```python
from build123d import *

# Parameters (mm, degrees)
PAD_DEPTH     = 16
SKETCH001_R   = 12
SKETCH001_R_2 = 15
POCKET_DEPTH  = 20


with BuildPart() as part:
    # Sketch → Pad (new body)
    with BuildSketch(Plane.YZ):
        Polygon((0, 0), (0, 116), (500, 116), (500, 0), (250, 0), align=None)
    extrude(amount=-PAD_DEPTH)

    # Sketch001 (on Face7 of Pad) → Pocket (cut)
    with BuildSketch(Plane(origin=(-16, 0, 0), x_dir=(0, -1, 0), z_dir=(-1, 0, 0))):
        with Locations((-215, 73.70748)):
            Circle(SKETCH001_R)
        with Locations((-285, 73.70748)):
            Circle(SKETCH001_R)
        with Locations((-450, 50)):
            Circle(SKETCH001_R_2)
        with Locations((-50, 50)):
            Circle(SKETCH001_R_2)
    extrude(amount=-POCKET_DEPTH, mode=Mode.SUBTRACT)


solid = part.part
```
Geometry check sheet. Reference: the model listing, model coordinates, mm. Give positions to 0.01 mm unless a question says otherwise; leave off trailing zeros. Order: outer loops, then holes, each group sorted by start corner. A loop starts at its lowest first (then second) coordinate and runs counter-clockwise, first axis right, second up. Notation, with made-up numbers: (-18.5, -23.75) -> (21.5, -23.75) arc R14 ccw to (21.5, -17.75) -> close; hole circle Ø10 at (73, 78.5). An arc over 180 degrees is marked (long way). Write each question's results on one line, items separated by ' | '. Start each with the question number.
(1) Gauge pin test, flat end, axial feed: P1, Ø18, axis at y = 450, z = 50, coming from the +X side. Record the tip position at first contact, or that the pin passes through.
(2) Scan lines: line 1 (Y direction, x = -14, z = 72.5); line 2 (Z direction, x = -12.5, y = 50); line 3 (Y direction, x = -7, z = 63). Record each from-to range of solid material in increasing order.
(3) Mould release check, pull along Y, two halves, no side actions. Record for faces 1 (the face through (-8.112, 461.056, 60.138)), 2 (the face through (-8, 500, 59)), 3 (the face through (-16, 253, 59)): pulls with the +Y half, pulls with the -Y half, needs draft (parallel to the pull), parting line crosses it, or undercut.
(4) Sectioned sample at D-D (y = 50). Enter the section's corners in (x, z).
(5) Sectioned sample at C-C (x = -11). Enter the section's corners in (y, z).
(6) Sectioned sample at A-A (z = 50). Enter the section's corners in (x, y).
(7) Sectioned sample at B-B (y = 215). Enter the section's corners in (x, z), plus the area to 3 significant figures.
Answer below:
1) P1: through
2) line 1: 0 to 203.06, 226.94 to 273.06, 296.94 to 500 | line 2: 0 to 35, 65 to 116 | line 3: 0 to 42.52, 57.48 to 209.58, 220.42 to 279.58, 290.42 to 442.52, 457.48 to 500
3) face 1: undercut | face 2: pulls with the +Y half | face 3: needs draft
4) outline: (-16, 0) -> (0, 0) -> (0, 35) -> (-16, 35) -> close; (-16, 65) -> (0, 65) -> (0, 116) -> (-16, 116) -> close
5) outline: (0, 0) -> (500, 0) -> (500, 116) -> (0, 116) -> close; hole circle Ø30 at (50, 50); hole circle Ø24 at (215, 73.71); hole circle Ø24 at (285, 73.71); hole circle Ø30 at (450, 50)
6) outline: (-16, 0) -> (0, 0) -> (0, 35) -> (-16, 35) -> close; (-16, 65) -> (0, 65) -> (0, 435) -> (-16, 435) -> close; (-16, 465) -> (0, 465) -> (0, 500) -> (-16, 500) -> close
7) outline: (-16, 0) -> (0, 0) -> (0, 61.71) -> (-16, 61.71) -> close; (-16, 85.71) -> (0, 85.71) -> (0, 116) -> (-16, 116) -> close | area: 1,470 mm2
